Verification items for the finished model (mm, model axes). Face numbers are marked on the shaded views. A direction names the side the tool comes from. Coordinates: 2 decimals unless noted, no trailing zeros. Write each loop counter-clockwise with the first axis right and the second up, starting at its lowest first coordinate (ties: lowest second). Pieces come first, ordered by that corner, then holes. Notation, with made-up numbers: (-32.5, 19.25) -> (4.5, 19.25) arc R9 cw to (4.5, 26.25) -> close; hole circle Ø9 at (29.25, 47.5). An arc over 180 degrees is marked (long way). Use CSV: the item, a comma, the result in double quotes.
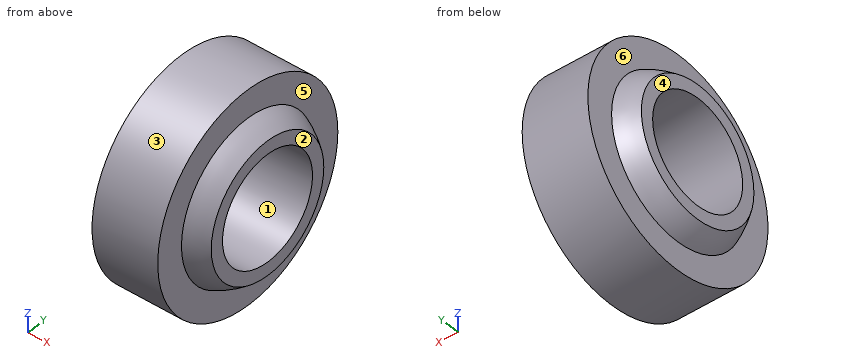
```python
from build123d import *


with BuildPart() as part:
    # 草图1 → 旋转1 (revolve)
    with BuildSketch(Plane.XY):
        with BuildLine():
            Line((4.4431655, 5.894913061), (4.4431655, 8))
            Line((4.4431655, 8), (-0.5568345, 8))
            Line((-0.5568345, 8), (-0.5568345, 5.894913061))
            ThreePointArc((-0.5568345, 5.894913061), (-1.337492566, 5.498843756), (-2.0568345, 5))
            Line((-2.0568345, 5), (-2.0568345, 4))
            Line((-2.0568345, 4), (5.9431655, 4))
            Line((5.9431655, 4), (5.9431655, 5))
            ThreePointArc((5.9431655, 5), (5.223823567, 5.498843756), (4.4431655, 5.894913061))
        make_face()
    revolve(axis=Axis((0, 0, 0), (1, 0, 0)))


solid = part.part
```
1) Cross-section at B-B (z = 1.75). Record the boundary of the cut face in (x, y).
Return value:
outline,"(-2.06, -4.68) arc R6.16 ccw to (-0.56, -5.63) -> (-0.56, -7.81) -> (4.44, -7.81) -> (4.44, -5.63) arc R6.16 ccw to (5.94, -4.68) -> (5.94, -3.6) -> (-2.06, -3.6) -> close; (-2.06, 3.6) -> (5.94, 3.6) -> (5.94, 4.68) arc R6.16 ccw to (4.44, 5.63) -> (4.44, 7.81) -> (-0.56, 7.81) -> (-0.56, 5.63) arc R6.16 ccw to (-2.06, 4.68) -> close"
2) Mould release check, pull along Y, two halves, no side actions. Record for the marked faces 1, 2 and 3: released by +Y, released by -Y, zero draft, split by the parting line, or undercut.
Return value:
face 1,"undercut"
face 2,"zero draft"
face 3,"split by the parting line"
3) Set-up check for the marked faces 4, 5 and 6: record each of +Z, -Z, +X, -X, +Y, -Y from which the full face is reachable in a straight line by a thin tool's end or side.
Return value:
face 4,"+Z, -Z, -X, +Y, -Y"
face 5,"+X"
face 6,"-X"
4) Scan lines: L1, parallel to Z at x = 0, y = 0; L2, parallel to X at y = -4, z = -5.5; L3, parallel to Y at x = 4, z = -0.5. Record each from-to range of solid material in increasing order.
Return value:
L1,"-8 to -4, 4 to 8"
L2,"-0.56 to 4.44"
L3,"-7.98 to -3.97, 3.97 to 7.98"
5) Gauge pin test, flat ends, axial feed: pin 1 (4 mm diameter, centred on x = 4, y = 3, fed in from +Z); pin 2 (1.5 mm diameter, centred on x = 2.5, y = -3.5, fed in from +Z); pin 3 (1 mm diameter, centred on x = 2.5, z = -1.5, fed in from -Y). Record the tip position at first contact, or that the pin passes through.
Return value:
pin 1,"z = 7.94"
pin 2,"z = 7.51"
pin 3,"y = -7.94"
6) Cross-section at C-C (x = 2.25). Record the boundary of the cut face in (y, z).
Return value:
outline,"circle Ø16 at (0, 0); hole circle Ø8 at (0, 0)"
7) Cross-section at D-D (y = 5.5). Record the boundary of the cut face in (x, z), plus the area to 3 significant figures.
Return value:
outline,"(-0.56, -5.81) -> (4.44, -5.81) -> (4.44, -2.12) arc R3.28 ccw to (4.44, 2.12) -> (4.44, 5.81) -> (-0.56, 5.81) -> (-0.56, 2.12) arc R3.28 ccw to (-0.56, -2.12) -> close"
area,"62.6 mm2"
8) Cross-section at A-A (y = 0). Record the boundary of the cut face in (x, z), plus the area to 3 significant figures.
Return value:
outline,"(-2.06, -5) arc R6.4 ccw to (-0.56, -5.89) -> (-0.56, -8) -> (4.44, -8) -> (4.44, -5.89) arc R6.4 ccw to (5.94, -5) -> (5.94, -4) -> (-2.06, -4) -> close; (-2.06, 4) -> (5.94, 4) -> (5.94, 5) arc R6.4 ccw to (4.44, 5.89) -> (4.44, 8) -> (-0.56, 8) -> (-0.56, 5.89) arc R6.4 ccw to (-2.06, 5) -> close"
area,"49.0 mm2"
